from build123d import *

# Parameters (mm, degrees)
SKETCH1_R           = 88.9
BOSS_EXTRUDE1_DEPTH = 25.4
SKETCH2_R           = 12.5
BOSS_EXTRUDE2_DEPTH = 10
FILLET1_R           = 5
SKETCH3_R           = 30
CUT_EXTRUDE1_DEPTH  = 129.263712717


with BuildPart() as part:
    # Sketch1 → Boss-Extrude1 (new body)
    with BuildSketch(Plane(origin=(0, 0, 0), x_dir=(1, 0, 0), z_dir=(0, 1, 0))):
        with Locations(Location((0, 0, 0), (0, 0, 270))):
            Circle(SKETCH1_R)
    extrude(amount=BOSS_EXTRUDE1_DEPTH)

    # Sketch2 → Boss-Extrude2 (add)
    with BuildSketch(Plane(origin=(0, 25.4, 0), x_dir=(1, 0, 0), z_dir=(0, 1, 0))):
        with Locations(Location((65, 0, 0), (0, 0, 270))):
            Circle(SKETCH2_R)
    extrude(amount=BOSS_EXTRUDE2_DEPTH)

    # Fillet1
    fillet1_edges = [part.edges().sort_by_distance(p)[0] for p in [
        (65, 25.4, -12.5),
        (65, 35.4, -12.5),
    ]]
    fillet(fillet1_edges, radius=FILLET1_R - 0.0001)  # a hair under: the kernel refuses the full size

    # Sketch3 → Cut-Extrude1 (cut, through all)
    with BuildSketch(Plane(origin=(0, 25.4, 0), x_dir=(1, 0, 0), z_dir=(0, 1, 0))):
        with Locations(Location((0, 0, 0), (0, 0, 270))):
            Circle(SKETCH3_R)
    extrude(amount=-CUT_EXTRUDE1_DEPTH, mode=Mode.SUBTRACT)


solid = part.part
Input: part model. Units: mm. Frame: model coordinates. Coordinates: 2 decimals unless noted, no trailing zeros. Loops run counter-clockwise (first coordinate to the right, second up) from the corner with the lowest first, then second, coordinate; pieces in that order, holes last.
(1) Section B-B on x = 0. Return the cut outline in (y, z).
(2) Section C-C on y = 15.5. Return the cut outline in (x, z), then the cut area to 3 significant figures.
(3) Material intervals for probe 1 along X at (y, z) = (19.25, 0); probe 2 along Y at (x, z) = (42.5, -59.5); probe 3 along X at (y, z) = (18, 23.5), sorted ascending.
(4) First-contact query: pin 1 Ø1.5 at (y, z) = (15, 35.5) entering from -X; pin 2 Ø3 at (x, y) = (53.5, 12.5) entering from -Z; pin 3 Ø3 at (x, y) = (39.5, 20) entering from -Z. Flat tips, straight axial feed; report the tip coordinate or a pass-through.
(5) Pull-direction query (X, two-part tool) for faces 1 (the face through (1.32, 12.88, -29.97)), 2 (the face through (-38, 25.4, -1)), 3 (the face through (74.96, 12.52, 47.79)); classes: released by +X, released by -X, zero draft, split by the parting line, or undercut.
Data:
1. outline: (0, -88.9) - (25.4, -88.9) - (25.4, -30) - (0, -30) - close; (0, 30) - (25.4, 30) - (25.4, 88.9) - (0, 88.9) - close
2. outline: circle Ø177.8 at (0, 0); hole circle Ø60 at (0, 0)
2. area: 22,000 mm2
3. probe 1: x = -88.9 to -30, 30 to 88.9
3. probe 2: y = 0 to 25.4
3. probe 3: x = -85.74 to -18.65, 18.65 to 85.74
4. pin 1: stops at x = -81.83
4. pin 2: stops at z = -72.11
4. pin 3: stops at z = -80.37
5. face 1: undercut
5. face 2: zero draft
5. face 3: split by the parting line
